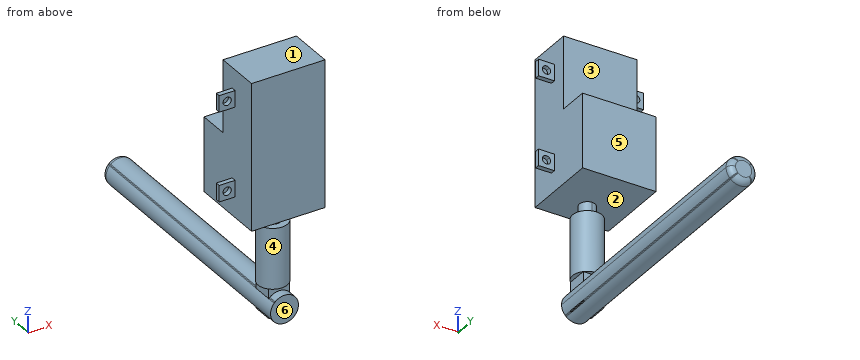
from build123d import *

# Parameters (mm, degrees)
SKETCH_1_W           = 5.4
SKETCH_1_H           = 5.6
SKETCH_1_R           = 1.4
EXTRUDE_1_DEPTH      = 1.6
EXTRUDE_2_DEPTH      = 5
EXTRUDE_3_DEPTH      = 9
SKETCH_5_W           = 25
SKETCH_5_H           = 25.3
EXTRUDE_4_DEPTH      = 10.4
EXTRUDE_5_DEPTH      = 4.43
SKETCH_7_R           = 5
EXTRUDE_6_DEPTH      = 20.58
SKETCH_8_W           = 7.087670288
SKETCH_8_H           = 7.054426262
EXTRUDE_7_DEPTH      = 10
EXTRUDE_8_DEPTH      = 82
EXTRUDE_8_DEPTH_BACK = 10
FILLET_1_R           = 2


with BuildPart() as part:
    # 草图1 → 凸台-拉伸1 (new body)
    # profile 1 of 12: a face of its own
    with BuildSketch(Plane(origin=(0, 0, 0), x_dir=(1, 0, 0), z_dir=(0, 1, 0))):
        Polygon((0, -25), (0, 25), (-12.5, 25), (-12.5, 18), (-12.5, 12.4), (-12.5, -12.4), (-12.5, -18), (-12.5, -25), align=None)
    # profile 2 of 12: a face of its own
    with BuildSketch(Plane(origin=(0, 0, 0), x_dir=(1, 0, 0), z_dir=(0, 1, 0))):
        Polygon((12.5, 18), (12.5, 25), (0, 25), (0, -25), (12.5, -25), (12.5, -18), (12.5, -12.4), (12.5, 12.4), align=None)
    # profile 3 of 12: a face of its own
    with BuildSketch(Plane(origin=(0, 0, 0), x_dir=(1, 0, 0), z_dir=(0, 1, 0))):
        with Locations((-15.2, -15.2)):
            Rectangle(SKETCH_1_W, SKETCH_1_H)
        with Locations(Location((-15.2, -15.2, 0), (0, 0, 270))):
            Circle(SKETCH_1_R, mode=Mode.SUBTRACT)
    # profile 4 of 12: a face of its own
    with BuildSketch(Plane(origin=(0, 0, 0), x_dir=(1, 0, 0), z_dir=(0, 1, 0))):
        with Locations((-15.2, 15.2)):
            Rectangle(SKETCH_1_W, SKETCH_1_H)
        with Locations(Location((-15.2, 15.2, 0), (0, 0, 270))):
            Circle(SKETCH_1_R, mode=Mode.SUBTRACT)
    # profile 5 of 12: a face of its own
    with BuildSketch(Plane(origin=(0, 0, 0), x_dir=(1, 0, 0), z_dir=(0, 1, 0))):
        with BuildLine():
            Line((14.228210201, 14.192217986), (12.5, 12.4))
            Line((12.5, 12.4), (17.9, 12.4))
            Line((17.9, 12.4), (16.171789799, 14.192217986))
            ThreePointArc((16.171789799, 14.192217986), (15.2, 13.8), (14.228210201, 14.192217986))
        make_face()
    # profile 6 of 12: a face of its own
    with BuildSketch(Plane(origin=(0, 0, 0), x_dir=(1, 0, 0), z_dir=(0, 1, 0))):
        with BuildLine():
            Line((17.9, 18), (12.5, 18))
            Line((12.5, 18), (14.228210201, 16.207782014))
            ThreePointArc((14.228210201, 16.207782014), (15.2, 16.6), (16.171789799, 16.207782014))
            Line((16.171789799, 16.207782014), (17.9, 18))
        make_face()
    # profile 7 of 12: a face of its own
    with BuildSketch(Plane(origin=(0, 0, 0), x_dir=(1, 0, 0), z_dir=(0, 1, 0))):
        with BuildLine():
            Line((17.9, 12.4), (17.9, 18))
            Line((17.9, 18), (16.171789799, 16.207782014))
            ThreePointArc((16.171789799, 16.207782014), (16.488507997, 15.747491681), (16.6, 15.2))
            ThreePointArc((16.6, 15.2), (16.488507997, 14.652508319), (16.171789799, 14.192217986))
            Line((16.171789799, 14.192217986), (17.9, 12.4))
        make_face()
    # profile 8 of 12: a face of its own
    with BuildSketch(Plane(origin=(0, 0, 0), x_dir=(1, 0, 0), z_dir=(0, 1, 0))):
        with BuildLine():
            Line((14.228210201, 16.207782014), (12.5, 18))
            Line((12.5, 18), (12.5, 12.4))
            Line((12.5, 12.4), (14.228210201, 14.192217986))
            ThreePointArc((14.228210201, 14.192217986), (13.8, 15.2), (14.228210201, 16.207782014))
        make_face()
    # profile 9 of 12: a face of its own
    with BuildSketch(Plane(origin=(0, 0, 0), x_dir=(1, 0, 0), z_dir=(0, 1, 0))):
        with BuildLine():
            Line((17.9, -12.4), (12.5, -12.4))
            Line((12.5, -12.4), (14.228210201, -14.192217986))
            ThreePointArc((14.228210201, -14.192217986), (15.2, -13.8), (16.171789799, -14.192217986))
            Line((16.171789799, -14.192217986), (17.9, -12.4))
        make_face()
    # profile 10 of 12: a face of its own
    with BuildSketch(Plane(origin=(0, 0, 0), x_dir=(1, 0, 0), z_dir=(0, 1, 0))):
        with BuildLine():
            Line((14.228210201, -14.192217986), (12.5, -12.4))
            Line((12.5, -12.4), (12.5, -18))
            Line((12.5, -18), (14.228210201, -16.207782014))
            ThreePointArc((14.228210201, -16.207782014), (13.8, -15.2), (14.228210201, -14.192217986))
        make_face()
    # profile 11 of 12: a face of its own
    with BuildSketch(Plane(origin=(0, 0, 0), x_dir=(1, 0, 0), z_dir=(0, 1, 0))):
        with BuildLine():
            Line((17.9, -18), (17.9, -12.4))
            Line((17.9, -12.4), (16.171789799, -14.192217986))
            ThreePointArc((16.171789799, -14.192217986), (16.488507997, -14.652508319), (16.6, -15.2))
            ThreePointArc((16.6, -15.2), (16.488507997, -15.747491681), (16.171789799, -16.207782014))
            Line((16.171789799, -16.207782014), (17.9, -18))
        make_face()
    # profile 12 of 12: a face of its own
    with BuildSketch(Plane(origin=(0, 0, 0), x_dir=(1, 0, 0), z_dir=(0, 1, 0))):
        with BuildLine():
            Line((14.228210201, -16.207782014), (12.5, -18))
            Line((12.5, -18), (17.9, -18))
            Line((17.9, -18), (16.171789799, -16.207782014))
            ThreePointArc((16.171789799, -16.207782014), (15.2, -16.6), (14.228210201, -16.207782014))
        make_face()
    extrude(amount=EXTRUDE_1_DEPTH)

    # 草图3 → 凸台-拉伸2 (add)
    with BuildSketch(Plane(origin=(0, 1.6, 0), x_dir=(1, 0, 0), z_dir=(0, 1, 0))):
        Polygon((12.5, 25), (-12.5, 25), (-12.5, 18), (-12.5, 12.4), (-12.5, -12.4), (-12.5, -18), (-12.5, -25), (12.5, -25), (12.5, -18), (12.5, -12.4), (12.5, 12.4), (12.5, 18), align=None)
    extrude(amount=EXTRUDE_2_DEPTH)

    # 草图4 → 凸台-拉伸3 (add)
    with BuildSketch(Plane.XZ):
        Polygon((12.5, 25), (-12.5, 25), (-12.5, 18), (-12.5, 12.4), (-12.5, -12.4), (-12.5, -18), (-12.5, -25), (12.5, -25), (12.5, -18), (12.5, -12.4), (12.5, 12.4), (12.5, 18), align=None)
    extrude(amount=EXTRUDE_3_DEPTH)

    # 草图5 → 凸台-拉伸4 (add)
    with BuildSketch(Plane(origin=(0, 6.6, 0), x_dir=(1, 0, 0), z_dir=(0, 1, 0))):
        with Locations((0, 12.35)):
            Rectangle(SKETCH_5_W, SKETCH_5_H)
    extrude(amount=EXTRUDE_4_DEPTH)

    # 草图6 → 凸台-拉伸5 (add)
    with BuildSketch(Plane(origin=(0, 0, -25), x_dir=(-1, 0, 0), z_dir=(0, 0, -1))):
        with BuildLine():
            ThreePointArc((0, 2.18), (-2.665, -0.485), (0, -3.15))
            Line((0, -3.15), (0, 2.18))
        make_face()
        with BuildLine():
            Line((0, 2.18), (0, -3.15))
            ThreePointArc((0, -3.15), (1.884439572, -2.369439572), (2.665, -0.485))
            ThreePointArc((2.665, -0.485), (1.884439572, 1.399439572), (0, 2.18))
        make_face()
    extrude(amount=EXTRUDE_5_DEPTH)

    # 草图7 → 凸台-拉伸6 (add)
    with BuildSketch(Plane(origin=(0, 0, -29.43), x_dir=(-1, 0, 0), z_dir=(0, 0, -1))):
        with Locations((0, -0.485)):
            Circle(SKETCH_7_R)
    extrude(amount=EXTRUDE_6_DEPTH)

    # 草图8 → 凸台-拉伸7 (add)
    with BuildSketch(Plane(origin=(0, 0, -50.01), x_dir=(-1, 0, 0), z_dir=(0, 0, -1))):
        with Locations((0, -0.485)):
            Rectangle(SKETCH_8_W, SKETCH_8_H)
    extrude(amount=EXTRUDE_7_DEPTH)

    # 草图9 → 凸台-拉伸8 (add, two sides: drawn at the far end of the back side and taken through both)
    with BuildSketch(Plane(origin=(0, 3.042213131, 0), x_dir=(1, 0, 0), z_dir=(0, 1, 0)).offset(-EXTRUDE_8_DEPTH_BACK)):
        with BuildLine():
            Line((3.543835144, 59.627867761), (3.543835144, 53.302132239))
            ThreePointArc((3.543835144, 53.302132239), (4.438226951, 54.772474806), (4.75, 56.465))
            ThreePointArc((4.75, 56.465), (4.438226951, 58.157525194), (3.543835144, 59.627867761))
        make_face()
        with BuildLine():
            ThreePointArc((3.161562114, 60.01), (0, 61.215), (-3.161562114, 60.01))
            Line((-3.161562114, 60.01), (3.161562114, 60.01))
        make_face()
        with BuildLine():
            Line((-3.543835144, 53.302132239), (-3.543835144, 59.627867761))
            ThreePointArc((-3.543835144, 59.627867761), (-4.75, 56.465), (-3.543835144, 53.302132239))
        make_face()
        with BuildLine():
            ThreePointArc((-3.161562114, 52.92), (0, 51.715), (3.161562114, 52.92))
            Line((3.161562114, 52.92), (-3.161562114, 52.92))
        make_face()
        with BuildLine():
            Line((3.358205246, 53.105690915), (0, 56.465))
            Line((0, 56.465), (-3.358205246, 53.105690915))
            ThreePointArc((-3.358205246, 53.105690915), (-3.261205588, 53.011445582), (-3.161562114, 52.92))
            Line((-3.161562114, 52.92), (3.161562114, 52.92))
            ThreePointArc((3.161562114, 52.92), (3.261205588, 53.011445582), (3.358205246, 53.105690915))
        make_face()
        with BuildLine():
            Line((0, 56.465), (-3.358205246, 59.824309085))
            ThreePointArc((-3.358205246, 59.824309085), (-3.452417658, 59.727408974), (-3.543835144, 59.627867761))
            Line((-3.543835144, 59.627867761), (-3.543835144, 53.302132239))
            ThreePointArc((-3.543835144, 53.302132239), (-3.452417658, 53.202591026), (-3.358205246, 53.105690915))
            Line((-3.358205246, 53.105690915), (0, 56.465))
        make_face()
        with BuildLine():
            ThreePointArc((-3.161562114, 60.01), (-3.261205588, 59.918554418), (-3.358205246, 59.824309085))
            Line((-3.358205246, 59.824309085), (0, 56.465))
            Line((0, 56.465), (3.358205246, 59.824309085))
            ThreePointArc((3.358205246, 59.824309085), (3.261205588, 59.918554418), (3.161562114, 60.01))
            Line((3.161562114, 60.01), (-3.161562114, 60.01))
        make_face()
        with BuildLine():
            Line((3.358205246, 59.824309085), (0, 56.465))
            Line((0, 56.465), (3.358205246, 53.105690915))
            ThreePointArc((3.358205246, 53.105690915), (3.452417658, 53.202591026), (3.543835144, 53.302132239))
            Line((3.543835144, 53.302132239), (3.543835144, 59.627867761))
            ThreePointArc((3.543835144, 59.627867761), (3.452417658, 59.727408974), (3.358205246, 59.824309085))
        make_face()
    extrude(amount=EXTRUDE_8_DEPTH + EXTRUDE_8_DEPTH_BACK)

    # 圆角1
    fillet_1_edges = [part.edges().sort_by_distance(p)[0] for p in [
        (-3.359309085, 85.042213131, -53.106794754),
    ]]
    fillet(fillet_1_edges, radius=FILLET_1_R)


solid = part.part
Model file for the job. Use its own axes, mm. Face numbers are marked on the shaded views. A direction names the side the tool comes from. Give positions to 0.01 mm unless a question says otherwise; leave off trailing zeros. Loops run counter-clockwise (first coordinate to the right, second up) from the corner with the lowest first, then second, coordinate; pieces in that order, holes last.
1) Tool access for the marked faces 4, 5 and 6: list every direction of +Z, -Z, +X, -X, +Y, -Y with a clear straight run to the whole face (end or side of a thin tool).
2) Saw through at A-A (x = -15.2). Write the cut outline in (y, z), plus the area to 3 significant figures.
3) Pull direction Z, two halves, no side cores. Call the marked faces 1, 2 and 3: +Z half, -Z half, draft (parallel to the pull), parting line (faces both ways), or undercut.
4) Saw through at C-C (x = -9). Write the cut outline in (y, z).
5) Saw through at B-B (y = 60). Write the cut outline in (x, z) (3 decimals).
6) Flat gauge pins, fed straight in: pin 1 Ø7.5 at (x, z) = (-5, 13.5) entering from +Y; pin 2 Ø1.2 at (x, y) = (4.5, 0.5) entering from -Z; pin 3 Ø3.5 at (y, z) = (-1.5, -52) entering from +X. Where does each tip first touch, or does it go through?
7) Saw through at D-D (z = -28). Write the cut outline in (x, y) (3 decimals).
8) Wall check: line 1 (X direction, y = 0.95, z = -15.2); line 2 (Y direction, x = 5.5, z = -5); line 3 (Z direction, x = 1, y = 8.5). Give the ranges that are in metal, low to high.
Answer block:
1. face 4: none
1. face 5: +Z, +X, -X, +Y
1. face 6: -Z, +X, -X, -Y
2. outline: (0, -18) - (1.6, -18) - (1.6, -16.6) - (0, -16.6) - close; (0, -13.8) - (1.6, -13.8) - (1.6, -12.4) - (0, -12.4) - close; (0, 12.4) - (1.6, 12.4) - (1.6, 13.8) - (0, 13.8) - close; (0, 16.6) - (1.6, 16.6) - (1.6, 18) - (0, 18) - close
2. area: 8.96 mm2
3. face 1: +Z half
3. face 2: undercut
3. face 3: draft
4. outline: (-9, -25) - (17, -25) - (17, 0.3) - (6.6, 0.3) - (6.6, 25) - (-9, 25) - close
5. outline: (-3.544, -53.302) arc R4.75 ccw to (-3.358, -59.824) arc R4.75 ccw to (-3.162, -60.01) arc R4.75 ccw to (3.358, -59.824) arc R4.75 ccw to (3.544, -59.628) arc R4.75 ccw to (3.358, -53.106) arc R4.75 ccw to (3.162, -52.92) arc R4.75 ccw to (-3.358, -53.106) arc R4.75 ccw to start
6. pin 1: stops at y = 6.6
6. pin 2: stops at z = -59.18
6. pin 3: stops at x = 3.9
7. outline: circle Ø5.33 at (0, -0.485)
8. line 1: x = -17.9 to -16.6, -13.8 to 13.8, 16.6 to 17.9
8. line 2: y = -9 to 17
8. line 3: z = -61.11 to -51.82, -25 to 0.3
